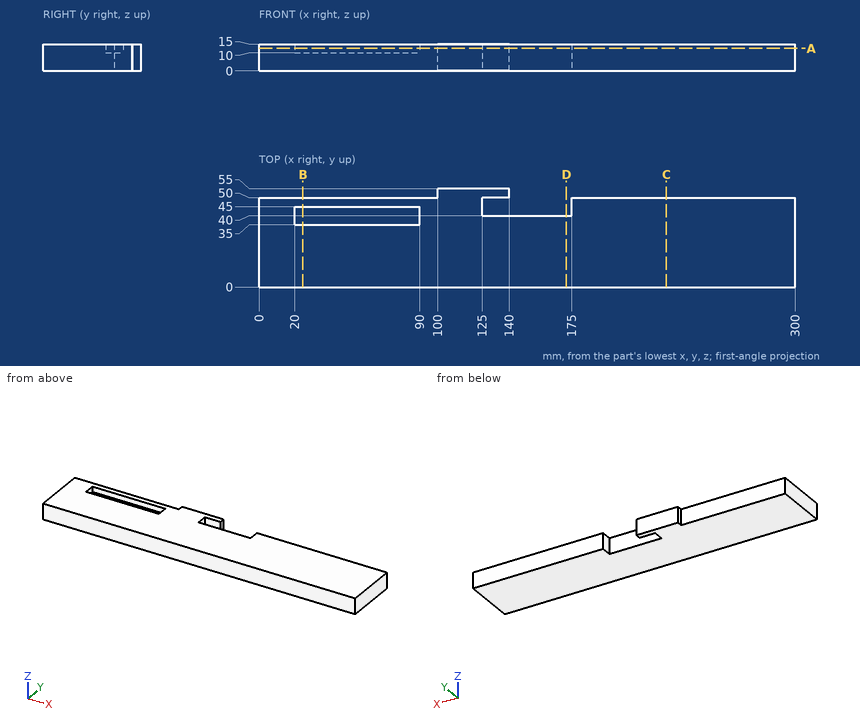
Print and shaded views of the part. All mm, measured from the part's lowest x, y and z. Round coordinates to 2 decimals unless told otherwise and drop trailing zeros. Write each loop counter-clockwise with the first axis right and the second up, starting at its lowest first coordinate (ties: lowest second). Pieces come first, ordered by that corner, then holes. Notation, with made-up numbers: M -8,33 L 38,33 A15 cw 38,58 Z; hole C 57,35.25 d4. An arc over 180 degrees is marked long. One line per question, with ' | ' between items.
(1) Saw through at C-C on x = 228. Write the cut outline in (y, z).
Answer key:
outline: M 0,0 L 50,0 L 50,15 L 0,15 Z
(2) Probe line 1 along Y through (x, z) = (58, 12); line 2 along X through (y, z) = (47.5, 7.25); line 3 along Y through (x, z) = (219, 6). List the from-to ranges inside material, lowest first.
Answer key:
line 1: y = 0 to 35, 45 to 50 | line 2: x = 0 to 125, 175 to 300 | line 3: y = 0 to 50
(3) Saw through at B-B on x = 24.5. Write the cut outline in (y, z), then the cut area to 3 significant figures.
Answer key:
outline: M 0,0 L 50,0 L 50,15 L 45,15 L 45,10 L 35,10 L 35,15 L 0,15 Z | area: 700 mm^2
(4) Saw through at D-D on x = 172. Write the cut outline in (y, z).
Answer key:
outline: M 0,0 L 40,0 L 40,15 L 0,15 Z
(5) Saw through at A-A on z = 12.5. Write the cut outline in (x, y), then the cut area to 3 significant figures.
Answer key:
outline: M 0,0 L 300,0 L 300,50 L 175,50 L 175,40 L 125,40 L 125,50 L 140,50 L 140,55 L 100,55 L 100,50 L 0,50 Z; hole M 20,35 L 90,35 L 90,45 L 20,45 Z | area: 14,000 mm^2
(6) Pin check, flat tips, straight feed: pin 1 (5 mm diameter, centred on x = 55.5, y = 40.5, fed in from +Z); pin 2 (1.5 mm diameter, centred on x = 246, z = 12, fed in from -Y); pin 3 (2 mm diameter, centred on x = 144.5, z = 13, fed in from +Y); pin 4 (5 mm diameter, centred on x = 219, z = 6, fed in from +Y). Stop position of each tip, or through.
Answer key:
pin 1: stops at z = 10 | pin 2: stops at y = 0 | pin 3: stops at y = 40 | pin 4: stops at y = 50
